Input: dimensioned drawing with shaded views. Units: mm. Origin: part minimum x, y, z. A direction names the side the tool comes from. Give positions to 0.01 mm unless a question says otherwise; leave off trailing zeros. Write each loop counter-clockwise with the first axis right and the second up, starting at its lowest first coordinate (ties: lowest second). Pieces come first, ordered by that corner, then holes. Notation, with made-up numbers: (15, 84) -> (19, 84) arc R20 cw to (19, 116) -> close; hole circle Ø8 at (17, 12). An arc over 180 degrees is marked (long way). Answer as a JSON object with one key per item and string values. Group by question number.
(1) Draft query along Z for the marked faces 1, 2 and 3. Return one class per face: +Z half, -Z half, draft (parallel to the pull), parting line (faces both ways), or undercut.
(2) Section query D-D on x = 4.75. Output: boundary loops of the cut face in (y, z), plus the area to 3 significant figures.
(3) Section query A-A on y = 11. Output: boundary loops of the cut face in (x, z).
(4) Set-up query: the marked faces 4 and 5. Return all of +Z, -Z, +X, -X, +Y, -Y with unobstructed straight access to the full face (end or side cutting, diameter ignored); none if empty.
(5) Section query B-B on z = 2.2. State how many separate pieces and enclosed holes the cut face has, plus the area to 3 significant figures.
(6) Contact query for flat-ended pins moving along their axis: pin 1 Ø4.5 at (x, y) = (7.04, 11.82) entering from +Z; pin 2 Ø1.5 at (y, z) = (3, 2) entering from -X; pin 3 Ø3 at (x, z) = (4, 1) entering from +Y; pin 4 Ø1.5 at (y, z) = (10.5, 1) entering from -X. Output: stop coordinate, or through.
(7) Section query C-C on y = 8.25. Output: boundary loops of the cut face in (x, z).
(8) Material intervals for probe 1 along Y at (x, z) = (7, 2.85) (1 decimal); probe 2 along Y at (x, z) = (7.75, 1.5) (1 decimal); probe 3 along X at (y, z) = (14, 0.8), sorted ascending.
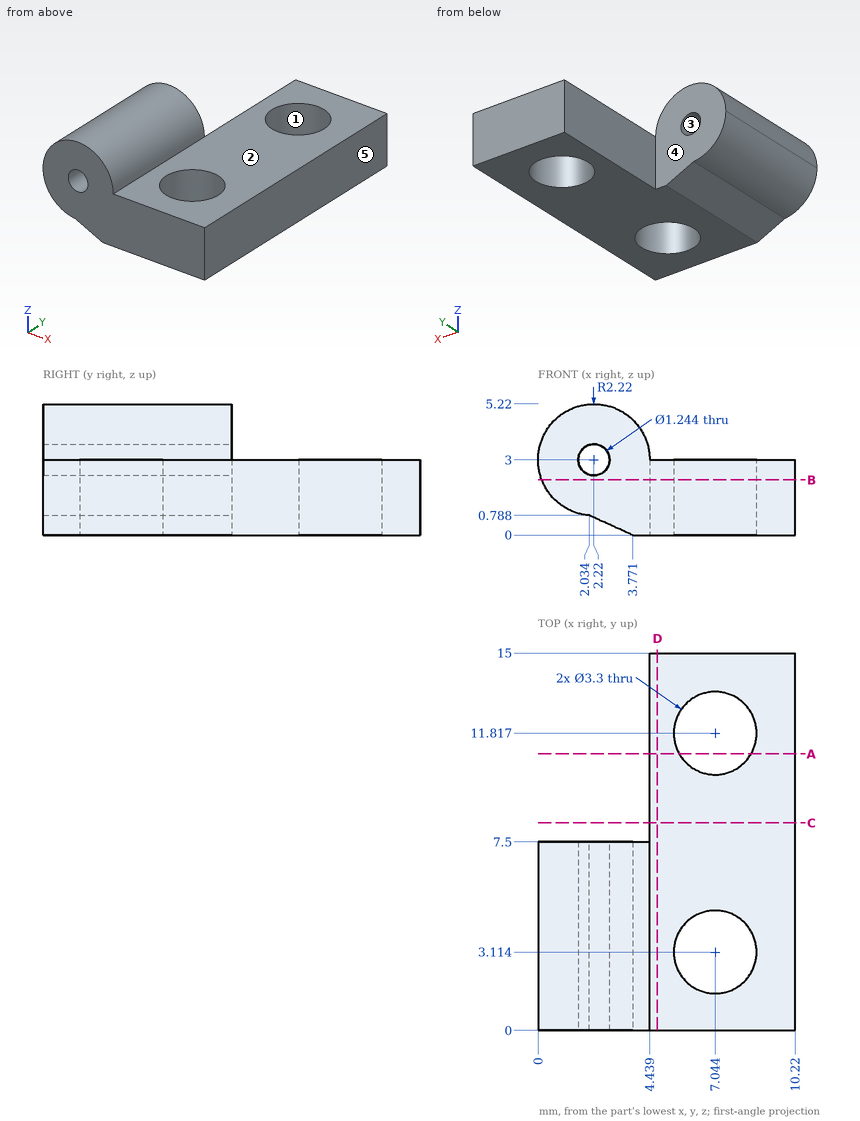
Answer list:
{
 "1": {"face 1": "draft", "face 2": "+Z half", "face 3": "undercut"},
 "2": {"outline": "(0, 0) -> (15, 0) -> (15, 3) -> (0, 3) -> close", "area": "45.0 mm2"},
 "3": {"outline": "(4.44, 0) -> (5.61, 0) -> (5.61, 3) -> (4.44, 3) -> close; (8.48, 0) -> (10.22, 0) -> (10.22, 3) -> (8.48, 3) -> close"},
 "4": {"face 4": "+Z, -Z, -X, +Y", "face 5": "+Z, -Z, +X, +Y, -Y"},
 "5": {"separate pieces": "1", "enclosed holes": "2", "area": "102 mm2"},
 "6": {"pin 1": "z = 3", "pin 2": "x = 0.01", "pin 3": "y = 15", "pin 4": "x = 4.44"},
 "7": {"outline": "(4.44, 0) -> (10.22, 0) -> (10.22, 3) -> (4.44, 3) -> close"},
 "8": {"probe 1": "0 to 1.5, 4.8 to 10.2, 13.5 to 15", "probe 2": "0 to 1.6, 4.6 to 10.3, 13.3 to 15", "probe 3": "4.44 to 10.22"}
}
